Geometry: final body of the model. Coordinates: model frame, mm. Face numbers are marked on the shaded views. A direction names the side the tool comes from. Coordinates: 2 decimals unless noted, no trailing zeros. Write each loop counter-clockwise with the first axis right and the second up, starting at its lowest first coordinate (ties: lowest second). Pieces come first, ordered by that corner, then holes.
from build123d import *

# Parameters (mm, degrees)
F0_R     = 9.5
F0_W     = 25
F0_H     = 23
F1_DEPTH = 55
F2_R     = 4
F3_DEPTH = 20
F4_R     = 1.5
F5_DEPTH = 3
F6_DEPTH = 55


with BuildPart() as f1:
    # F0 (on Front) → F1 (new body)
    with BuildSketch(Plane.XZ):
        Polygon((0, 4.9239983139), (-25, 4.9239983139), (-25, -25.0760016861), (10, -25.0760016861), (10, 4.9239983139), align=None)
        with Locations((-5, -10.0760016861)):
            Circle(F0_R, mode=Mode.SUBTRACT)
        with Locations((-12.5, 16.4239983139)):
            Rectangle(F0_W, F0_H)
    extrude(amount=F1_DEPTH)

    # F2 (on face) → F3 (cut)
    with BuildSketch(Plane(origin=(-25, 0, 0), x_dir=(0, -1, 0), z_dir=(-1, 0, 0))):
        with Locations((12, 12.9239983139)):
            Circle(F2_R)
        with Locations((43, 12.9239983139)):
            Circle(F2_R)
    extrude(amount=-F3_DEPTH, mode=Mode.SUBTRACT)

    # F4 (on face) → F5 (cut)
    with BuildSketch(Plane(origin=(0, 0, -25.0760016861), x_dir=(1, 0, 0), z_dir=(0, 0, -1))):
        Polygon((-17, 29.2320508076), (-20, 30.9641016151), (-23, 29.2320508076), (-23, 25.7679491924), (-20, 24.0358983849), (-17, 25.7679491924), align=None)
        with Locations((-20, 27.5)):
            Circle(F4_R, mode=Mode.SUBTRACT)
    extrude(amount=-F5_DEPTH, mode=Mode.SUBTRACT)

    # F6 (cut): a face of the model
    f6_faces = [f1.faces().sort_by_distance(p)[0] for p in [
        (-20, -27.5, -25.0760016861),
    ]]
    extrude(f6_faces, amount=-F6_DEPTH, mode=Mode.SUBTRACT)


solid = f1.part
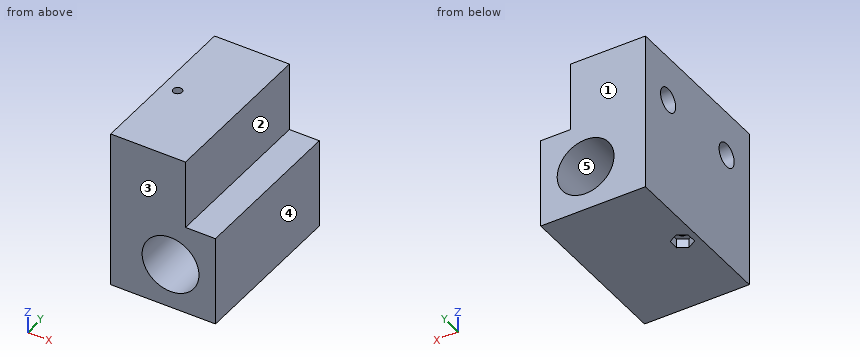
Item 1: Section D-D, the plane z = 18. Output: boundary loops of the cut face in (x, y), plus the area to 3 significant figures.
Derived:
outline: (-25, -55) - (0, -55) - (0, 0) - (-25, 0) - close; hole circle Ø3 at (-20, -27.5)
area: 1,370 mm2
Item 2: Section A-A, the plane z = -7. Output: boundary loops of the cut face in (x, y), plus the area to 3 significant figures.
Derived:
outline: (-25, -55) - (-13.99, -55) - (-13.99, 0) - (-25, 0) - close; (3.99, -55) - (10, -55) - (10, 0) - (3.99, 0) - close; hole circle Ø3 at (-20, -27.5)
area: 929 mm2
Item 3: Material intervals for probe 1 along Y at (x, z) = (-20, 7); probe 2 along Z at (x, y) = (-10.25, -12); probe 3 along Z at (x, y) = (-9, -43), sorted ascending.
Derived:
probe 1: y = -55 to -29, -26 to 0
probe 2: z = -25.08 to -17.99, -2.16 to 8.92, 16.92 to 27.92
probe 3: z = -25.08 to -18.69, -1.46 to 8.92, 16.92 to 27.92
Item 4: Pin query (flat end, axial travel): pin 1 (5 mm diameter, centred on y = -12, z = 12.92, fed in from +X); pin 2 (3 mm diameter, centred on x = 3.5, y = -31.5, fed in from +Z); pin 3 (2.5 mm diameter, centred on y = -42, z = 13, fed in from -X). Return the tip coordinate at first contact, or that it passes through.
Derived:
pin 1: stops at x = 0
pin 2: stops at z = 4.92
pin 3: stops at x = -5
Item 5: Pull-direction query (X, two-part tool) for the marked faces 3, 4 and 5; classes: released by +X, released by -X, zero draft, split by the parting line, or undercut.
Derived:
face 3: zero draft
face 4: released by +X
face 5: undercut
Item 6: Section B-B, the plane y = -27.5. Output: boundary loops of the cut face in (x, z).
Derived:
outline: (-25, -25.08) - (-23, -25.08) - (-23, -22.08) - (-21.5, -22.08) - (-21.5, 27.92) - (-25, 27.92) - close; (-18.5, -22.08) - (-17, -22.08) - (-17, -25.08) - (10, -25.08) - (10, 4.92) - (0, 4.92) - (0, 27.92) - (-18.5, 27.92) - close; hole circle Ø19 at (-5, -10.08)
Item 7: Set-up query: the marked faces 1 and 2. Return all of +Z, -Z, +X, -X, +Y, -Y with unobstructed straight access to the full face (end or side cutting, diameter ignored); none if empty.
Derived:
face 1: +Z, -Z, +X, -X, +Y
face 2: +Z, +X, +Y, -Y
Item 8: Section C-C, the plane y = -9. Output: boundary loops of the cut face in (x, z).
Derived:
outline: (-25, -25.08) - (10, -25.08) - (10, 4.92) - (0, 4.92) - (0, 27.92) - (-25, 27.92) - (-25, 15.57) - (-5, 15.57) - (-5, 10.28) - (-25, 10.28) - close; hole circle Ø19 at (-5, -10.08)
